from build123d import *

# Parameters (mm, degrees)
F2_DEPTH = 40
F3_DEPTH = 50
F5_D     = 20


with BuildPart() as f2:
    # F0 (on Front) → F2 (new body, symmetric)
    with BuildSketch(Plane.XZ):
        with BuildLine():
            Line((-74.1799686244, 44.5079811746), (-74.1799686244, -44.5079811746))
            Line((-74.1799686244, -44.5079811746), (74.1799686244, -44.5079811746))
            Line((74.1799686244, -44.5079811746), (74.1799686244, 44.5079811746))
            Line((74.1799686244, 44.5079811746), (49.1799686244, 44.5079811746))
            ThreePointArc((49.1799686244, 44.5079811746), (0, -4.6719874497), (-49.1799686244, 44.5079811746))
            Line((-49.1799686244, 44.5079811746), (-74.1799686244, 44.5079811746))
        make_face()
    extrude(amount=F2_DEPTH, both=True)

    # F1 (on Front) → F3 (join, symmetric)
    with BuildSketch(Plane.XZ):
        with BuildLine():
            Line((-35.1070836186, 44.7443202138), (-49.149915576, 44.7443202138))
            ThreePointArc((-49.149915576, 44.7443202138), (-1.8626e-06, -5.0042579476), (49.1499118507, 44.7443202138))
            Line((49.1499118507, 44.7443202138), (35.3824310005, 44.7443202138))
            ThreePointArc((35.3824310005, 44.7443202138), (0.1376736909, 9.1714728244), (-35.1070836186, 44.7443202138))
        make_face()
    extrude(amount=F3_DEPTH, both=True)

    # F5 (through all)
    with Locations(Plane(origin=(0, 0, -44.5079811746), x_dir=(1, 0, 0), z_dir=(0, 0, -1))):
        with Locations((-61.6649421002, 0), (61.6649402375, 0)):
            Hole(F5_D / 2)


solid = f2.part
Part model, mm, in its own coordinate system. A direction names the side the tool comes from. Coordinates: 2 decimals unless noted, no trailing zeros. Loops run counter-clockwise (first coordinate to the right, second up) from the corner with the lowest first, then second, coordinate; pieces in that order, holes last. Notation, with made-up numbers: (87, 61) - (130, 61) arc R14 cw to (130, 81) - close; hole circle Ø11 at (69.25, 9.5). An arc over 180 degrees is marked (long way). Write each question's results on one line, items separated by ' | '. Start each with the question number.
Q1. Probe line 1 along X through (y, z) = (-7.5, -2); line 2 along Y through (x, z) = (-38.5, -28); line 3 along X through (y, z) = (-28, 23.5). List the from-to ranges inside material, lowest first.
Q2. Slice it at C-C on z = 25. Give the cut face in (x, y), and give its area (3 significant figures).
Q3. Which spindle directions (+Z, -Z, +X, -X, +Y, -Y) get a long thin tool onto all of the face, cutting with end or side? Do faces 1 (the flat face through (-56, -9, 44.508)), 2 (the flat face through (-1, 50, 9)), 3 (the cylindrical face through (-6.111, 40.507, -4.623)), 4 (the flat face through (-1, -40, -9)), 5 (the flat face through (-1, 40, -9)). Say none if no direction does.
Q4. Slice it at D-D on z = 7. Give the cut face in (x, y), and give its area (3 significant figures).
Q5. Slice it at A-A on y = 0. Give the cut face in (x, z).
Q6. Two-plate mould, pull along X, no slides. Class faces 6 (the flat face through (74.18, -1, -1)), 7 (the flat face through (67, -9, 44.508)), 8 (the cylindrical face through (0.92, -0.7, 9.18)): +X half, -X half, draft (parallel to the pull), parting line (faces both ways), or undercut.
Q7. Slice it at B-B on x = 62. Give the cut face in (y, z).
Q8. Drop flat-ended pins along their axis: pin 1 Ø8 at (x, z) = (47.5, -4) entering from -Y; pin 2 Ø8 at (x, z) = (50.5, -28.5) entering from +Y; pin 3 Ø7.5 at (x, y) = (67.5, 3) entering from +Z. Give the stop position or say it passes through.
Answer:
1) line 1: x = -74.18 to -68.28, -55.05 to 55.05, 68.28 to 74.18 | line 2: y = -40 to 40 | line 3: x = -74.18 to -28.23, 28.51 to 74.18
2) outline: (-74.18, -40) - (-45.27, -40) - (-45.27, -50) - (-29.28, -50) - (-29.28, 50) - (-45.27, 50) - (-45.27, 40) - (-74.18, 40) - close; (29.55, -50) - (45.27, -50) - (45.27, -40) - (74.18, -40) - (74.18, 40) - (45.27, 40) - (45.27, 50) - (29.55, 50) - close; hole circle Ø20 at (-61.66, 0); hole circle Ø20 at (61.66, 0) | area: 7,170 mm2
3) face 1: +Z, -X, +Y, -Y | face 2: +Z, -Z, +X, -X, +Y | face 3: none | face 4: -Z, -Y | face 5: -Z, +Y
4) outline: (-74.18, -40) - (-32.19, -40) - (-32.19, -50) - (32.19, -50) - (32.19, -40) - (74.18, -40) - (74.18, 40) - (32.19, 40) - (32.19, 50) - (-32.19, 50) - (-32.19, 40) - (-74.18, 40) - close; hole circle Ø20 at (-61.66, 0); hole circle Ø20 at (61.66, 0) | area: 12,500 mm2
5) outline: (-74.18, -44.51) - (-71.66, -44.51) - (-71.66, 44.51) - (-74.18, 44.51) - close; (-51.66, -44.51) - (51.66, -44.51) - (51.66, 44.51) - (49.18, 44.51) arc R49.18 cw to (49.03, 40.7) arc R49.15 ccw to (49.15, 44.74) - (35.38, 44.74) arc R35.25 cw (long way) to (-35.11, 44.74) - (-49.15, 44.74) arc R49.15 ccw to (-49.03, 40.7) arc R49.18 cw to (-49.18, 44.51) - (-51.66, 44.51) - close; (71.66, -44.51) - (74.18, -44.51) - (74.18, 44.51) - (71.66, 44.51) - close
6) face 6: +X half | face 7: draft | face 8: undercut
7) outline: (-40, -44.51) - (-9.99, -44.51) - (-9.99, 44.51) - (-40, 44.51) - close; (9.99, -44.51) - (40, -44.51) - (40, 44.51) - (9.99, 44.51) - close
8) pin 1: stops at y = -40 | pin 2: stops at y = 40 | pin 3: stops at z = 44.51
